CAD build for the part. Positions are in the model's coordinates, mm. Coordinates: 2 decimals unless noted, no trailing zeros. Write each loop counter-clockwise with the first axis right and the second up, starting at its lowest first coordinate (ties: lowest second). Pieces come first, ordered by that corner, then holes. Notation, with made-up numbers: M 60.25,-2 L 81.25,-2 A24 cw 81.25,8 Z; hole C 9.25,37 d2. An arc over 180 degrees is marked long. Answer as CSV lines item,"result". Start each with the question number.
```python
from build123d import *

# Parameters (mm, degrees)
F0_R     = 1.5875
F1_DEPTH = 7.9502


with BuildPart() as f1:
    # F0 (on Front) → F1 (new body)
    with BuildSketch(Plane.XZ):
        with BuildLine():
            Line((0, 12.0413007322), (0, 37.4413007322))
            ThreePointArc((0, 37.4413007322), (-6.7801009863, 40.2763189971), (-9.5241473512, 47.0937457472))
            Line((-9.5241473512, 47.0937457472), (-15.7480782934, -1.8302884103))
            ThreePointArc((-15.7480782934, -1.8302884103), (-10.4931281713, 8.0788943281), (0, 12.0413007322))
        make_face()
        with Locations((-6.5820463933, 33.9521430433)):
            Circle(F0_R, mode=Mode.SUBTRACT)
        with BuildLine():
            ThreePointArc((9.525, 46.9663007322), (6.7351920908, 40.2311086414), (0, 37.4413007322))
            Line((0, 37.4413007322), (0, 12.0413007322))
            ThreePointArc((0, 12.0413007322), (10.5003255158, 8.0725507322), (15.7504882737, -1.8493242678))
            Line((15.7504882737, -1.8493242678), (9.4502929642, 48.1569257322))
            ThreePointArc((9.4502929642, 48.1569257322), (9.5063048942, 47.5627839741), (9.525, 46.9663007322))
        make_face()
        with BuildLine():
            ThreePointArc((-9.5241473512, 47.0937457472), (-6.7801009863, 40.2763189971), (0, 37.4413007322))
            ThreePointArc((0, 37.4413007322), (6.7351920908, 40.2311086414), (9.525, 46.9663007322))
            ThreePointArc((9.525, 46.9663007322), (9.5063048942, 47.5627839741), (9.4502929642, 48.1569257322))
            ThreePointArc((9.4502929642, 48.1569257322), (-0.5328710329, 56.4763834585), (-9.5241473512, 47.0937457472))
        make_face()
        with BuildLine():
            ThreePointArc((3.175, 46.9663007322), (2.2450640303, 44.7212367019), (0, 43.7913007322))
            ThreePointArc((0, 43.7913007322), (-2.2450640303, 49.2113647624), (3.175, 46.9663007322))
        make_face(mode=Mode.SUBTRACT)
        with BuildLine():
            ThreePointArc((15.7504882737, -1.8493242678), (10.5003255158, 8.0725507322), (0, 12.0413007322))
            Line((0, 12.0413007322), (0, 3.175))
            ThreePointArc((0, 3.175), (2.2450640303, 2.2450640303), (3.175, 0))
            ThreePointArc((3.175, 0), (2.2450640303, -2.2450640303), (0, -3.175))
            Line((0, -3.175), (0, -19.7086992678))
            ThreePointArc((0, -19.7086992678), (9.4368838065, -16.5993112399), (15.1770200819, -8.4891999321))
            ThreePointArc((15.1770200819, -8.4891999321), (15.6995353243, -6.1874655265), (15.875, -3.8336992678))
            ThreePointArc((15.875, -3.8336992678), (15.8438414904, -2.8395605312), (15.7504882737, -1.8493242678))
        make_face()
        with BuildLine():
            Line((0, 3.175), (0, 12.0413007322))
            ThreePointArc((0, 12.0413007322), (-10.4931281713, 8.0788943281), (-15.7480782934, -1.8302884103))
            ThreePointArc((-15.7480782934, -1.8302884103), (-11.9125935959, -14.3268274391), (0, -19.7086992678))
            Line((0, -19.7086992678), (0, -3.175))
            ThreePointArc((0, -3.175), (-3.175, 0), (0, 3.175))
        make_face()
        with BuildLine():
            ThreePointArc((0, -19.7086992678), (-11.9125935959, -14.3268274391), (-15.7480782934, -1.8302884103))
            Line((-15.7480782934, -1.8302884103), (-16.0137054558, -3.9182859294))
            Line((-16.0137054558, -3.9182859294), (-9.4762655267, -68.2959968664))
            ThreePointArc((-9.4762655267, -68.2959968664), (-7.067231057, -60.9477874154), (0, -57.8086992678))
            Line((0, -57.8086992678), (0, -19.7086992678))
        make_face()
        with BuildLine():
            ThreePointArc((15.1770200819, -8.4891999321), (9.4368838065, -16.5993112399), (0, -19.7086992678))
            Line((0, -19.7086992678), (0, -57.8086992678))
            ThreePointArc((0, -57.8086992678), (6.7351920908, -60.598507177), (9.525, -67.3336992678))
            Line((9.525, -67.3336992678), (41.8581225716, -67.3336992678))
            ThreePointArc((41.8581225716, -67.3336992678), (44.2728781992, -61.6325414164), (50.0479054623, -59.4002095191))
            Line((50.0479054623, -59.4002095191), (17.2861640166, -58.3583947443))
            ThreePointArc((17.2861640166, -58.3583947443), (11.470504938, -55.5484416885), (9.6601438639, -49.3484159244))
            Line((9.6601438639, -49.3484159244), (15.1770200819, -8.4891999321))
        make_face()
        with BuildLine():
            Line((41.8581225716, -67.3336992678), (9.525, -67.3336992678))
            ThreePointArc((9.525, -67.3336992678), (6.9458584111, -73.8514194163), (0.6051730325, -76.8394549243))
            Line((0.6051730325, -76.8394549243), (50.0479054623, -75.2671890166))
            ThreePointArc((50.0479054623, -75.2671890166), (44.2728781992, -73.0348571193), (41.8581225716, -67.3336992678))
        make_face()
        with BuildLine():
            Line((0, -64.1586992678), (0, -57.8086992678))
            ThreePointArc((0, -57.8086992678), (-7.067231057, -60.9477874154), (-9.4762655267, -68.2959968664))
            ThreePointArc((-9.4762655267, -68.2959968664), (-6.3859118524, -74.4009303248), (0, -76.8586992678))
            Line((0, -76.8586992678), (0.6051730325, -76.8394549243))
            ThreePointArc((0.6051730325, -76.8394549243), (6.9458584111, -73.8514194163), (9.525, -67.3336992678))
            Line((9.525, -67.3336992678), (3.175, -67.3336992678))
            ThreePointArc((3.175, -67.3336992678), (-2.2450640303, -69.5787632981), (0, -64.1586992678))
        make_face()
        with BuildLine():
            ThreePointArc((9.525, -67.3336992678), (6.7351920908, -60.598507177), (0, -57.8086992678))
            Line((0, -57.8086992678), (0, -64.1586992678))
            ThreePointArc((0, -64.1586992678), (2.2450640303, -65.0886352376), (3.175, -67.3336992678))
            Line((3.175, -67.3336992678), (9.525, -67.3336992678))
        make_face()
        with BuildLine():
            ThreePointArc((50.0479054623, -59.4002095191), (44.2728781992, -61.6325414164), (41.8581225716, -67.3336992678))
            ThreePointArc((41.8581225716, -67.3336992678), (44.2728781992, -73.0348571193), (50.0479054623, -75.2671890166))
            ThreePointArc((50.0479054623, -75.2671890166), (55.4967804231, -72.8564436402), (57.7331225716, -67.3336992678))
            ThreePointArc((57.7331225716, -67.3336992678), (55.4967804231, -61.8109548955), (50.0479054623, -59.4002095191))
        make_face()
        with BuildLine():
            ThreePointArc((52.9706225716, -67.3336992678), (49.7956225716, -70.5086992678), (46.6206225716, -67.3336992678))
            ThreePointArc((46.6206225716, -67.3336992678), (49.7956225716, -64.1586992678), (52.9706225716, -67.3336992678))
        make_face(mode=Mode.SUBTRACT)
    extrude(amount=F1_DEPTH)


solid = f1.part
```
1) Band-saw the part on A-A, the plane y = -5. State how many separate pieces and enclosed holes the cut face has, plus the area to 3 significant figures.
2) Probe L1, parallel to Z at x = 1.5, y = -0.5; L2, parallel to Z at x = -5.5, y = -2.75; L3, parallel to X at y = -6, z = 38. List the from-to ranges inside material, lowest first. Write a range as [from, to].
3) Band-saw the part on C-C, the plane z = -17.5. List the corners of the cut face in (x, y), plus the area to 3 significant figures.
4) Two-plate mould, pull along X, no slides. Class faces 1 (the cylindrical face through (-7.75, -3.92, 35.03)), 2 (the cylindrical face through (48.33, -3.92, -70.15)), 3 (the flat face through (12.38, -3.92, -29.2)), 4 (the cylindrical face through (-6.458, -3.919, -74.335)): pulls with the +X half, pulls with the -X half, needs draft (parallel to the pull), parting line crosses it, or undercut.
5) Pin check, flat tips, straight feed: P1, Ø2, axis at x = 18, y = -6, coming from the -Z side; P2, Ø2, axis at x = 10, y = -2.5, coming from the -Z side; P3, Ø2, axis at y = -4.5, z = -14.5, coming from the -X side. Stop position of each tip, or through.
6) Band-saw the part on B-B, the plane x = 29.5. List the corners of the cut face in (y, z).
Result sheet:
1,separate pieces,"1"
1,enclosed holes,"5"
1,area,"3,840 mm²"
2,L1,"z = [-76.81, -70.13], [-64.54, -2.8], [2.8, 44.17], [49.76, 56.37]"
2,L2,"z = [-75.11, 32.79], [35.11, 54.74]"
2,L3,"x = [-10.68, 10.73]"
3,outline,"M -14.63,-7.95 L 13.96,-7.95 L 13.96,0 L -14.63,0 Z"
3,area,"227 mm²"
4,face 1,"undercut"
4,face 2,"undercut"
4,face 3,"pulls with the +X half"
4,face 4,"pulls with the -X half"
5,P1,"stops at z = -76.32"
5,P2,"stops at z = -76.57"
5,P3,"stops at x = -15.04"
6,outline,"M -7.95,-75.92 L 0,-75.92 L 0,-58.75 L -7.95,-58.75 Z"
